from build123d import *

# Parameters (mm, degrees)
SKETCH2_W           = 150
SKETCH2_H           = 120
BOSS_EXTRUDE1_DEPTH = 20
FILLET1_R           = 10
BOSS_EXTRUDE2_DEPTH = 10
CUT_EXTRUDE1_DEPTH  = 30
CUT_EXTRUDE2_DEPTH  = 15


with BuildPart() as part:
    # Sketch2 → Boss-Extrude1 (new body)
    with BuildSketch(Plane(origin=(0, 0, 0), x_dir=(1, 0, 0), z_dir=(0, 1, 0))):
        Rectangle(SKETCH2_W, SKETCH2_H)
    extrude(amount=BOSS_EXTRUDE1_DEPTH)

    # Fillet1
    fillet1_edges = [part.edges().sort_by_distance(p)[0] for p in [
        (-75, 20, 0),
        (0, 20, 60),
        (75, 20, 0),
        (75, 10, 60),
        (-75, 10, 60),
        (-75, 10, -60),
        (75, 10, -60),
        (0, 20, -60),
    ]]
    fillet(fillet1_edges, radius=FILLET1_R)

    # Sketch3 → Boss-Extrude2 (add)
    with BuildSketch(Plane.XZ):
        with BuildLine():
            ThreePointArc((-64.75, 39.75), (-61.821067812, 46.821067812), (-54.75, 49.75))
            Line((-54.75, 49.75), (54.75, 49.75))
            ThreePointArc((54.75, 49.75), (61.821067812, 46.821067812), (64.75, 39.75))
            Line((64.75, 39.75), (64.75, -39.75))
            ThreePointArc((64.75, -39.75), (61.821067812, -46.821067812), (54.75, -49.75))
            Line((54.75, -49.75), (-54.75, -49.75))
            ThreePointArc((-54.75, -49.75), (-61.821067812, -46.821067812), (-64.75, -39.75))
            Line((-64.75, -39.75), (-64.75, 39.75))
        make_face()
    extrude(amount=BOSS_EXTRUDE2_DEPTH)

    # Sketch4 → Cut-Extrude1 (cut)
    with BuildSketch(Plane(origin=(0, 20, 0), x_dir=(1, 0, 0), z_dir=(0, 1, 0))):
        with BuildLine():
            Line((52.5, -38.5), (52.5, -43))
            ThreePointArc((52.5, -43), (56.5, -47), (60.5, -43))
            Line((60.5, -43), (60.5, 44))
            ThreePointArc((60.5, 44), (56.5, 48), (52.5, 44))
            Line((52.5, 44), (52.5, 39.5))
            Line((52.5, 39.5), (-52.5, 39.5))
            Line((-52.5, 39.5), (-52.5, 44))
            ThreePointArc((-52.5, 44), (-56.5, 48), (-60.5, 44))
            Line((-60.5, 44), (-60.5, -43.000001))
            ThreePointArc((-60.5, -43.000001), (-56.5, -47.000001), (-52.5, -43.000001))
            Line((-52.5, -43.000001), (-52.5, -38.5))
            Line((-52.5, -38.5), (52.5, -38.5))
        make_face()
    extrude(amount=-CUT_EXTRUDE1_DEPTH, mode=Mode.SUBTRACT)

    # Sketch4<3> → Cut-Extrude2 (cut)
    with BuildSketch(Plane(origin=(0, 20, 0), x_dir=(1, 0, 0), z_dir=(0, 1, 0))):
        with BuildLine():
            Line((-50, -43.000001), (-50, -41))
            Line((-50, -41), (50, -41))
            Line((50, -41), (50, -43))
            ThreePointArc((50, -43), (56.5, -49.5), (63, -43))
            Line((63, -43), (63, 44))
            ThreePointArc((63, 44), (61.908326913, 47.605551275), (59, 50))
            Line((59, 50), (54, 50))
            ThreePointArc((54, 50), (51.091673087, 47.605551275), (50, 44))
            Line((50, 44), (50, 42))
            Line((50, 42), (-50, 42))
            Line((-50, 42), (-50, 44))
            ThreePointArc((-50, 44), (-51.091673087, 47.605551275), (-54, 50))
            Line((-54, 50), (-59, 50))
            ThreePointArc((-59, 50), (-61.908326913, 47.605551275), (-63, 44))
            Line((-63, 44), (-63, -43.000001))
            ThreePointArc((-63, -43.000001), (-56.5, -49.500001), (-50, -43.000001))
        make_face()
        with BuildLine():
            Line((52.5, 39.5), (52.5, 44))
            ThreePointArc((52.5, 44), (56.5, 48), (60.5, 44))
            Line((60.5, 44), (60.5, -43))
            ThreePointArc((60.5, -43), (56.5, -47), (52.5, -43))
            Line((52.5, -43), (52.5, -38.5))
            Line((52.5, -38.5), (-52.5, -38.5))
            Line((-52.5, -38.5), (-52.5, -43.000001))
            ThreePointArc((-52.5, -43.000001), (-56.5, -47.000001), (-60.5, -43.000001))
            Line((-60.5, -43.000001), (-60.5, 44))
            ThreePointArc((-60.5, 44), (-56.5, 48), (-52.5, 44))
            Line((-52.5, 44), (-52.5, 39.5))
            Line((-52.5, 39.5), (52.5, 39.5))
        make_face(mode=Mode.SUBTRACT)
    extrude(amount=-CUT_EXTRUDE2_DEPTH, mode=Mode.SUBTRACT)


solid = part.part
Input: part model. Units: mm. Frame: model coordinates. A direction names the side the tool comes from. Coordinates: 2 decimals unless noted, no trailing zeros. Write each loop counter-clockwise with the first axis right and the second up, starting at its lowest first coordinate (ties: lowest second). Pieces come first, ordered by that corner, then holes. Notation, with made-up numbers: M 63,59.5 L 88,59.5 A34 cw 88,91.5 Z; hole C -2,43 d11. An arc over 180 degrees is marked long. Answer as a JSON object with one key per item and string values. Group by question number.
(1) Contact query for flat-ended pins moving along their axis: P1, Ø1.5, axis at x = 56, y = 14.5, coming from the +Z side; P2, Ø3, axis at y = -5, z = -33.5, coming from the +X side; P3, Ø2, axis at y = 15.5, z = 42.5, coming from the +X side; P4, Ø3, axis at x = -57.5, z = -6.5, coming from the +Y side. Output: stop coordinate, or through.
(2) Section D-D on y = 13.25. Output: boundary loops of the cut face in (x, z).
(3) Set-up query: faces 1 (the face through (57, 13, -50)), 2 (the face through (-1, -2, 38.5)), 3 (the face through (61.74, -4.93, 46.9)). Return all of +Z, -Z, +X, -X, +Y, -Y with unobstructed straight access to the full face (end or side cutting, diameter ignored); none if empty.
(4) Mould query, pull axis Z, two halves, no side actions, for faces 4 (the face through (56.6, -2.4, -48)), 5 (the face through (-61.74, -4.93, -46.9)), 6 (the face through (51.12, 12.6, -47.65)), 7 (the face through (-61.9, -4.93, 46.74)). Classes: pulls with the +Z half, pulls with the -Z half, needs draft (parallel to the pull), parting line crosses it, or undercut.
(5) Section C-C on y = -3. Output: boundary loops of the cut face in (x, z).
(6) Section B-B on x = -38. Output: boundary loops of the cut face in (y, z).
(7) Section A-A on z = -36. Output: boundary loops of the cut face in (x, y).
(8) Ray query, line 1 along Z through (x, y) = (-22, 5.75); line 2 along X through (y, z) = (14.25, -46.5); line 3 along X through (y, z) = (1.25, -28.5). Return the intervals inside material, ascending. Write a range as [from, to].
Result set:
{
 "1": {"P1": "stops at z = 59.27", "P2": "stops at x = 64.75", "P3": "stops at x = 73.93", "P4": "passes through"},
 "2": {"outline": "M -74.46,-50 A9.46 ccw -65,-59.46 L 65,-59.46 A9.46 ccw 74.46,-50 L 74.46,50 A9.46 ccw 65,59.46 L -65,59.46 A9.46 ccw -74.46,50 Z; hole M -63,-44 A6.5 ccw -59,-50 L -54,-50 A6.5 ccw -50,-44 L -50,-42 L 50,-42 L 50,-44 A6.5 ccw 54,-50 L 59,-50 A6.5 ccw 63,-44 L 63,43 A6.5 ccw 50,43 L 50,41 L -50,41 L -50,43 A6.5 ccw -63,43 Z"},
 "3": {"face 1": "+Y", "face 2": "+Y, -Y", "face 3": "+Z, +X, -Y"},
 "4": {"face 4": "undercut", "face 5": "pulls with the -Z half", "face 6": "undercut", "face 7": "pulls with the +Z half"},
 "5": {"outline": "M -64.75,-39.75 A10 ccw -54.75,-49.75 L 54.75,-49.75 A10 ccw 64.75,-39.75 L 64.75,39.75 A10 ccw 54.75,49.75 L -54.75,49.75 A10 ccw -64.75,39.75 Z; hole M -60.5,-44 A4 ccw -52.5,-44 L -52.5,-39.5 L 52.5,-39.5 L 52.5,-44 A4 ccw 60.5,-44 L 60.5,43 A4 ccw 52.5,43 L 52.5,38.5 L -52.5,38.5 L -52.5,43 A4 ccw -60.5,43 Z"},
 "6": {"outline": "M -10,-49.75 L 0,-49.75 L 0,-60 L 10,-60 A10 ccw 20,-50 L 20,-42 L 5,-42 L 5,-39.5 L -10,-39.5 Z; M -10,38.5 L 5,38.5 L 5,41 L 20,41 L 20,50 A10 ccw 10,60 L 0,60 L 0,49.75 L -10,49.75 Z"},
 "7": {"outline": "M -75,0 L -64.75,0 L -64.75,-10 L -60.5,-10 L -60.5,5 L -63,5 L -63,20 L -65,20 A10 ccw -75,10 Z; M 60.5,-10 L 64.75,-10 L 64.75,0 L 75,0 L 75,10 A10 ccw 65,20 L 63,20 L 63,5 L 60.5,5 Z"},
 "8": {"line 1": "z = [-60, -42], [41, 60]", "line 2": "x = [-74.05, -62.5], [-50.5, 50.5], [62.5, 74.05]", "line 3": "x = [-75, -60.5], [60.5, 75]"}
}
